Answer from the drawing. Dimensions are ordinates in mm from the lowest x, y and z of the part. A direction names the side the tool comes from. Give positions to 0.01 mm unless a question says otherwise; leave off trailing zeros. Write each loop counter-clockwise with the first axis right and the second up, starting at its lowest first coordinate (ties: lowest second). Pieces come first, ordered by that corner, then holes.
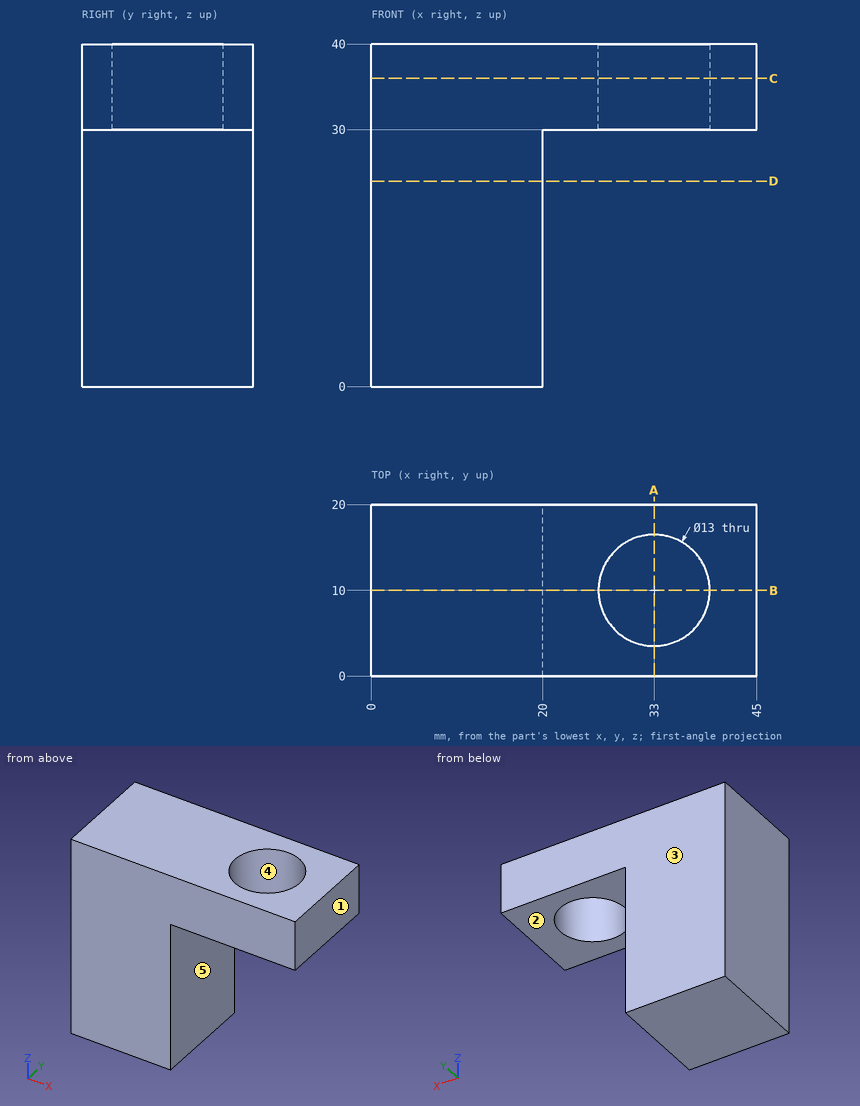
Item 1: Consider probe 1 along Y at (x, z) = (33, 34); probe 2 along X at (y, z) = (12.5, 35.5); probe 3 along X at (y, z) = (4.75, 31). Determine where each line is inside the solid, lowest interval first.
Conclusion:
probe 1: y = 0 to 3.5, 16.5 to 20
probe 2: x = 0 to 27, 39 to 45
probe 3: x = 0 to 29.17, 36.83 to 45
Item 2: A cutting plane is placed at A-A, the plane x = 33. Give the vertices of the cut face in (y, z).
Conclusion:
outline: (0, 30) - (3.5, 30) - (3.5, 40) - (0, 40) - close; (16.5, 30) - (20, 30) - (20, 40) - (16.5, 40) - close
Item 3: A cutting plane is placed at C-C, the plane z = 36. Give the vertices of the cut face in (x, y).
Conclusion:
outline: (0, 0) - (45, 0) - (45, 20) - (0, 20) - close; hole circle Ø13 at (33, 10)
Item 4: A cutting plane is placed at D-D, the plane z = 24. Give the vertices of the cut face in (x, y).
Conclusion:
outline: (0, 0) - (20, 0) - (20, 20) - (0, 20) - close
Item 5: Each of these flat-tipped pins is pushed along its axis until it touches: P1, Ø10, axis at x = 34, y = 6, coming from the -Z side; P2, Ø12, axis at y = 18, z = 11, coming from the +X side. Where does it stop, or does it pass through?
Conclusion:
P1: stops at z = 30
P2: stops at x = 20
Item 6: Determine the mould class of the marked faces 3, 4 and 5 for opening direction X: pulls with the +X half, pulls with the -X half, needs draft (parallel to the pull), parting line crosses it, or undercut.
Conclusion:
face 3: needs draft
face 4: undercut
face 5: pulls with the +X half
Item 7: A cutting plane is placed at B-B, the plane y = 10. Give the vertices of the cut face in (x, z).
Conclusion:
outline: (0, 0) - (20, 0) - (20, 30) - (26.5, 30) - (26.5, 40) - (0, 40) - close; (39.5, 30) - (45, 30) - (45, 40) - (39.5, 40) - close
Item 8: Which of the six approach directions +Z, -Z, +X, -X, +Y, -Y give full straight-line access (tool end or side, diameter ignored) to the marked faces 1 and 2?
Conclusion:
face 1: +Z, -Z, +X, +Y, -Y
face 2: -Z, +X, +Y, -Y
